Can you work these out from the model? Positions are in its coordinate system, mm. A direction names the side the tool comes from. Round coordinates to 2 decimals unless told otherwise and drop trailing zeros. Order: outer loops, then holes, each group sorted by start corner. A loop starts at its lowest first (then second) coordinate and runs counter-clockwise, first axis right, second up.
Q1. For faces 1 (the face through (11.5, 0, 10)), 2 (the face through (-11.5, 0, 25)), 3 (the face through (3.592, -0.097, 30.176)), 4 (the face through (11.5, 0, 25)), which set-ups out of +Z, -Z, +X, -X, +Y, -Y let a thin tool reach every point of the face, with its end or its side?
Q2. We'd pull the mould along Y, two halves only. Please class faces 5 (the face through (10.409, 1.915, 27.993)), 6 (the face through (-14, 0, 20.5)), 7 (the face through (12.76, 4.16, 21.24)): pulls with the +Y half, pulls with the -Y half, needs draft (parallel to the pull), parting line crosses it, or undercut.
Q3. If we section it at C-C (x = 5.79): Please give me the cut outline in (y, z).
Q4. If we section it at B-B (y = -4): Please give me the cut outline in (x, z).
Q5. Will these pins go through, and if not, where does the flat tip stop? P1, Ø1.3, axis at x = 13, y = 2.5, coming from the +Z side; P2, Ø3, axis at y = 3, z = 12, coming from the -X side; P3, Ø6, axis at y = 0, z = 12.5, coming from the +X side.
Q6. If we section it at A-A (x = -14): Please give me the cut outline in (y, z).
Q7. If I drill on line 1 (X direction, y = 4, z = 21.65); line 2 (Y direction, x = -14, z = 20.95); line 3 (X direction, y = 0, z = 5.5), over which ranges is the centre line in solid material (lowest first)?
Q8. If we section it at D-D (y = 0): Please give me the cut outline in (x, z).
Autodesk Inventor part; units mm, degrees
ref_plane "YZ Plane" through (0, 0, 0) normal (1, 0, 0) x (0, 1, 0)
ref_plane "XZ Plane" through (0, 0, 0) normal (0, 1, 0) x (-1, 0, 0)
ref_plane "XY Plane" through (0, 0, 0) normal (0, 0, 1) x (1, 0, 0)
sketch "スケッチ1" plane through (0, 0, 0) normal (0, 0, 1) x (1, 0, 0)
  line L0 (11.5, 6) -> (-11.5, 6)
  line L1 (-11.5, 6) -> (-11.5, -6)
  line L2 (-11.5, -6) -> (11.5, -6)
  line L3 (11.5, -6) -> (11.5, 6)
  line L4 (11.5, 6) -> (-11.5, -6) construction
  line L5 (-11.5, 6) -> (11.5, -6) construction
  point P0 (0, 0)
  dimension "d0" = 23
  dimension "d1" = 12
extrude "押し出し1" add sketch "スケッチ1" along normal blind 20.5
sketch "スケッチ2" plane through (0, 0, 20.5) normal (0, 0, 1) x (1, 0, 0)
  line L0 (-16, 6) -> (16, 6)
  line L1 (16, 6) -> (16, -6)
  line L2 (16, -6) -> (-16, -6)
  line L3 (-16, -6) -> (-16, 6)
  line L4 (-16, 6) -> (16, -6) construction
  line L5 (16, 6) -> (-16, -6) construction
  point P0 (0, 0)
  dimension "d4" = 32
  dimension "d5" = 12
extrude "押し出し2" add sketch "スケッチ2" along normal blind 1.5
sketch "スケッチ3" plane through (0, 0, 22) normal (0, 0, 1) x (1, 0, 0)
  line L0 (-11.5, 6) -> (-11.5, -6)
  line L1 (11.5, 6) -> (-11.5, 6)
  line L2 (11.5, -6) -> (11.5, 6)
  line L3 (-11.5, -6) -> (11.5, -6)
  point P0 (0, 0)
extrude "押し出し3" add sketch "スケッチ3" along normal blind 5.5
sketch "スケッチ4" plane through (0, 0, 27.5) normal (0, 0, 1) x (1, 0, 0)
  circle A0 centre (5.79, 0) radius 5
  line L0 (11.5, -6) -> (11.5, 6)
  line L1 (11.5, 6) -> (-11.5, 6)
  point P0 (0, 0)
  dimension "d10" = 5.71
  dimension "d11" = 6
  dimension "d12" = 10
extrude "押し出し4" add sketch "スケッチ4" along normal blind 1
sketch "スケッチ5" plane through (5.79, 0, 28.5) normal (0, 0, 1) x (1, 0, 0)
  circle A0 centre (0, 0) radius 5
  circle A1 centre (0, 0) radius 2.2
  point P0 (-5.79, 0)
  dimension "d15" = 4.4
extrude "押し出し5" add sketch "スケッチ5" along normal blind 3.4 contours A1
sketch "スケッチ6" plane through (0, 0, 22) normal (0, 0, 1) x (1, 0, 0)
  line L0 (-19.7007, 0) -> (19.7007, 0)
  line L1 (0, -8.8838) -> (0, 8.8838)
  circle A0 centre (5.79, 0) radius 2.2
  circle A1 centre (5.79, 0) radius 2.2
  line L2 (-11.5, 6) -> (-16, 6)
  line L3 (16, 6) -> (11.5, 6)
  point P0 (0, 0)
  point P1 (-14, 4)
  point P2 (-14, -4)
  point P3 (14, 4)
  point P4 (14, -4)
  dimension "d18" = 19.79
  dimension "d19" = 2
  dimension "d20" = 8.21
  dimension "d21" = 2
hole "穴1" at (-14, 4, 22) at (-14, -4, 22) at (14, 4, 22) at (14, -4, 22) direction (0, 0, -1) diameter 2.5 end through all
properties part number "STS3032"
Solution:
1. face 1: -Z, +X, +Y, -Y
1. face 2: +Z, -X, +Y, -Y
1. face 3: +Z
1. face 4: +Z, +X, +Y, -Y
2. face 5: parting line crosses it
2. face 6: needs draft
2. face 7: undercut
3. outline: (-6, 0) - (6, 0) - (6, 27.5) - (5, 27.5) - (5, 28.5) - (2.2, 28.5) - (2.2, 31.9) - (-2.2, 31.9) - (-2.2, 28.5) - (-5, 28.5) - (-5, 27.5) - (-6, 27.5) - close
4. outline: (-16, 20.5) - (-15.25, 20.5) - (-15.25, 22) - (-16, 22) - close; (-12.75, 20.5) - (-11.5, 20.5) - (-11.5, 0) - (11.5, 0) - (11.5, 20.5) - (12.75, 20.5) - (12.75, 22) - (11.5, 22) - (11.5, 27.5) - (8.79, 27.5) - (8.79, 28.5) - (2.79, 28.5) - (2.79, 27.5) - (-11.5, 27.5) - (-11.5, 22) - (-12.75, 22) - close; (15.25, 20.5) - (16, 20.5) - (16, 22) - (15.25, 22) - close
5. P1: stops at z = 22
5. P2: stops at x = -11.5
5. P3: stops at x = 11.5
6. outline: (-6, 20.5) - (-5.25, 20.5) - (-5.25, 22) - (-6, 22) - close; (-2.75, 20.5) - (2.75, 20.5) - (2.75, 22) - (-2.75, 22) - close; (5.25, 20.5) - (6, 20.5) - (6, 22) - (5.25, 22) - close
7. line 1: x = -16 to -15.25, -12.75 to 12.75, 15.25 to 16
7. line 2: y = -6 to -5.25, -2.75 to 2.75, 5.25 to 6
7. line 3: x = -11.5 to 11.5
8. outline: (-16, 20.5) - (-11.5, 20.5) - (-11.5, 0) - (11.5, 0) - (11.5, 20.5) - (16, 20.5) - (16, 22) - (11.5, 22) - (11.5, 27.5) - (10.79, 27.5) - (10.79, 28.5) - (7.99, 28.5) - (7.99, 31.9) - (3.59, 31.9) - (3.59, 28.5) - (0.79, 28.5) - (0.79, 27.5) - (-11.5, 27.5) - (-11.5, 22) - (-16, 22) - close
